from build123d import *

# Parameters (mm, degrees)
RESSALTO_EXTRUS_O1_DEPTH = 15
CORTE_EXTRUS_O1_DEPTH    = 240
ESBO_O4_R                = 2
CORTE_EXTRUS_O3_DEPTH    = 6
CORTE_EXTRUS_O4_START    = -6
ESBO_O6_R                = 2
CORTE_EXTRUS_O4_DEPTH    = 6


with BuildPart() as part:
    # Esboço1 → Ressalto-extrusão1 (new body)
    with BuildSketch(Plane.XY):
        with BuildLine():
            Line((-7.5, 6.160254038), (-7.5, -2.5))
            ThreePointArc((-7.5, -2.5), (-6.035533906, -6.035533906), (-2.5, -7.5))
            Line((-2.5, -7.5), (6.160254038, -7.5))
            ThreePointArc((6.160254038, -7.5), (4.571067812, 4.571067812), (-7.5, 6.160254038))
        make_face()
    extrude(amount=RESSALTO_EXTRUS_O1_DEPTH)

    # Esboço2 → Corte-extrusão1 (cut)
    with BuildSketch(Plane.XY.offset(15)):
        with BuildLine():
            Line((-3, 3.922616289), (-3, -1.737383711))
            ThreePointArc((-3, -1.737383711), (-2.630188251, -2.630188251), (-1.737383711, -3))
            Line((-1.737383711, -3), (3.922616289, -3))
            ThreePointArc((3.922616289, -3), (1.78599112, 1.78599112), (-3, 3.922616289))
        make_face()
    extrude(amount=-CORTE_EXTRUS_O1_DEPTH, mode=Mode.SUBTRACT)

    # Esboço4 → Corte-extrusão3 (cut)
    with BuildSketch(Plane.XY.offset(15)):
        with Locations((-3.690848423, -3.690848423)):
            Circle(ESBO_O4_R)
        with Locations((-4.5, 3.922616289)):
            Circle(ESBO_O4_R)
        with Locations((3.922616289, -4.5)):
            Circle(ESBO_O4_R)
    extrude(amount=-CORTE_EXTRUS_O3_DEPTH, mode=Mode.SUBTRACT)

    # Esboço6 → Corte-extrusão4 (cut)
    with BuildSketch(Plane(origin=(0, 0, 0), x_dir=(-1, 0, 0), z_dir=(0, 0, -1)).offset(CORTE_EXTRUS_O4_START)):
        with Locations((4.5, 3.922616289)):
            Circle(ESBO_O6_R)
        with Locations((-3.922616289, -4.5)):
            Circle(ESBO_O6_R)
        with Locations((3.690848423, -3.690848423)):
            Circle(ESBO_O6_R)
    extrude(amount=CORTE_EXTRUS_O4_DEPTH, mode=Mode.SUBTRACT)


solid = part.part
Read the model definition and answer for the solid it produces. Units are mm, in the model's axes. A direction names the side the tool comes from. Round coordinates to 2 decimals unless told otherwise and drop trailing zeros. Loops run counter-clockwise (first coordinate to the right, second up) from the corner with the lowest first, then second, coordinate; pieces in that order, holes last.
Q1. Which of the six approach directions +Z, -Z, +X, -X, +Y, -Y give full straight-line access (tool end or side, diameter ignored) to faces 5 (the face through (-5, 4, 9)), 6 (the face through (0, -3, 8)), 7 (the face through (-7.5, 2, 7)), 8 (the face through (-5.05, -5.16, 3.04))?
Q2. Section D-D on x = -3.75 is taken. Write down the section's boundary in (y, z).
Q3. Section C-C on y = 5 is taken. Write down the section's boundary in (x, z) (3 decimals).
Q4. Consider probe 1 along X at (y, z) = (-5, 12); probe 2 along Z at (x, y) = (-3, 5); probe 3 along X at (y, z) = (-4.5, 12.1). Determine where each line is inside the solid, lowest interval first.
Q5. Each of these flat-tipped pins is pushed along its axis until it touches: pin 1 (1.2 mm diameter, centred on x = -4, y = -4.5, fed in from +Z); pin 2 (1 mm diameter, centred on y = 0, z = 5.5, fed in from +X); pin 3 (3 mm diameter, centred on x = -3.69, y = -3.69, fed in from -Z). Where does it stop, or does it pass through?
Q6. Section B-B on x = 3.5 is taken. Write down the section's boundary in (y, z).
Q7. Section A-A on z = 10 is taken. Write down the section's boundary in (x, y), and give its area (3 significant figures).
Q8. Determine the mould class of faces 1 (the face through (-0.1, -3.2, 0)), 2 (the face through (-6.39, 4.58, 3.04)), 3 (the face through (4, -4, 9)), 4 (the face through (-6.07, -6, 7.4)) for opening direction Y: released by +Y, released by -Y, zero draft, split by the parting line, or undercut.
Output:
1. face 5: +Z
1. face 6: +Z, -Z
1. face 7: +Z, -Z, -X, +Y, -Y
1. face 8: -Z
2. outline: (-7.34, 0) - (-5.69, 0) - (-5.69, 6) - (-1.69, 6) - (-1.69, 0) - (2.07, 0) - (2.07, 6) - (5.78, 6) - (5.78, 0) - (7.42, 0) - (7.42, 15) - (5.78, 15) - (5.78, 9) - (2.07, 9) - (2.07, 15) - (-1.69, 15) - (-1.69, 9) - (-5.69, 9) - (-5.69, 15) - (-7.34, 15) - close
3. outline: (-7.5, 0) - (-6.185, 0) - (-6.185, 6) - (-2.815, 6) - (-2.815, 0) - (4.114, 0) - (4.114, 15) - (-2.815, 15) - (-2.815, 9) - (-6.185, 9) - (-6.185, 15) - (-7.5, 15) - close
4. probe 1: x = -6.83 to -5.2, -2.18 to 1.99, 5.86 to 7.18
4. probe 2: z = 6 to 9
4. probe 3: x = -7.08 to -5.52, -1.86 to 1.92, 5.92 to 7.3
5. pin 1: stops at z = 9
5. pin 2: stops at x = 7.3
5. pin 3: stops at z = 6
6. outline: (-7.5, 0) - (-6.45, 0) - (-6.45, 6) - (-3, 6) - (-3, 9) - (-6.45, 9) - (-6.45, 15) - (-7.5, 15) - close; (-0.91, 0) - (5.5, 0) - (5.5, 15) - (-0.91, 15) - close
7. outline: (-7.5, -2.5) arc R5 ccw to (-2.5, -7.5) - (6.16, -7.5) arc R10 ccw to (-7.5, 6.16) - close; hole (-3, -1.81) arc R2 ccw (long way) to (-1.81, -3) arc R1.26 ccw to (-1.74, -3) - (2.6, -3) arc R2 ccw (long way) to (3.88, -2.5) arc R7.33 ccw to (-2.5, 3.88) arc R2 ccw (long way) to (-3, 2.6) - (-3, -1.74) arc R1.26 ccw to start
7. area: 121 mm2
8. face 1: zero draft
8. face 2: undercut
8. face 3: undercut
8. face 4: released by -Y
